CAD build for the part. Positions are in the model's coordinates, mm. A direction names the side the tool comes from. Coordinates: 2 decimals unless noted, no trailing zeros. Order: outer loops, then holes, each group sorted by start corner. A loop starts at its lowest first (then second) coordinate and runs counter-clockwise, first axis right, second up. Notation, with made-up numbers: (27.5, -30.5) - (83.5, -30.5) arc R19 ccw to (83.5, -5.5) - close; hole circle Ø3 at (-14, 84). An arc over 180 degrees is marked (long way). Return JSON: item names as keys, results as strings.
from build123d import *

# Parameters (mm, degrees)
F1_DEPTH = 88.9
F2_SIZE  = 5.08
F3_SIZE  = 5.08
F4_SIZE  = 5.08
F5_SIZE  = 5.08
F6_SIZE  = 5.08
F7_SIZE  = 5.08
F8_R     = 8.414365
F9_DEPTH = 101.6
F10_SIZE = 7.62


with BuildPart() as f1:
    # F0 (on Front) → F1 (new body)
    with BuildSketch(Plane.XZ):
        Polygon((-22.467206, -10.215149), (2.772436, -24.524237), (24.180665, -4.941663), (12.172037, 21.470121), (-16.657933, 18.210928), align=None)
    extrude(amount=F1_DEPTH)

    # F2
    f2_edges = [f1.edges().sort_by_distance(p)[0] for p in [
        (-9.847385, -88.9, -17.369693),
    ]]
    chamfer(f2_edges, length=F2_SIZE)

    # F3
    f3_edges = [f1.edges().sort_by_distance(p)[0] for p in [
        (-19.027823, -88.9, 6.614521),
    ]]
    chamfer(f3_edges, length=F3_SIZE)

    # F4
    f4_edges = [f1.edges().sort_by_distance(p)[0] for p in [
        (0.410862, -88.9, 20.140535),
    ]]
    chamfer(f4_edges, length=F4_SIZE)

    # F5
    f5_edges = [f1.edges().sort_by_distance(p)[0] for p in [
        (19.28175, -88.9, 5.833014),
    ]]
    chamfer(f5_edges, length=F5_SIZE)

    # F6
    f6_edges = [f1.edges().sort_by_distance(p)[0] for p in [
        (13.476551, -88.9, -14.73295),
    ]]
    chamfer(f6_edges, length=F6_SIZE)

    # F7
    f7_edges = [f1.edges().sort_by_distance(p)[0] for p in [
        (-19.562569, 0, 3.997889),
        (-2.242948, 0, 19.840525),
        (18.176351, 0, 8.264229),
        (13.476551, 0, -14.73295),
        (-9.847385, 0, -17.369693),
    ]]
    chamfer(f7_edges, length=F7_SIZE)

    # F8 (on face) → F9 (join)
    with BuildSketch(Plane.XZ.offset(88.9)):
        Circle(F8_R)
    extrude(amount=F9_DEPTH)

    # F10
    f10_edges = [f1.edges().sort_by_distance(p)[0] for p in [
        (-8.414365, -190.5, 0),
    ]]
    chamfer(f10_edges, length=F10_SIZE)


solid = f1.part
Item 1: Drop flat-ended pins along their axis: P1, Ø1, axis at x = -6.5, y = -32, coming from the -Z side; P2, Ø12, axis at x = -10, z = 6, coming from the -Y side; P3, Ø6, axis at x = 15.5, z = 2.5, coming from the -Y side. Give the stop position or say it passes through.
Findings below:
{"P1": "stops at z = -19.55", "P2": "stops at y = -185.63", "P3": "stops at y = -88.9"}
Item 2: Band-saw the part on A-A, the plane y = -127.5. List the corners of the cut face in (x, z), then the cut area to 3 significant figures.
Findings below:
{"outline": "circle Ø16.83 at (0, 0)", "area": "222 mm²"}
Item 3: Band-saw the part on B-B, the plane y = -28. List the corners of the cut face in (x, z), then the cut area to 3 significant figures.
Findings below:
{"outline": "(-22.47, -10.22) - (2.77, -24.52) - (24.18, -4.94) - (12.17, 21.47) - (-16.66, 18.21) - close", "area": "1,450 mm²"}
Item 4: Which spindle directions (+Z, -Z, +X, -X, +Y, -Y) get a long thin tool onto all of the face, cutting with end or side? Do faces 1 (the flat face through (-17.07, -2.58, 3.7)), 2 (the cylindrical face through (4.524, -135.232, 7.095)). Say none if no direction does.
Findings below:
{"face 1": "+Z, -X, +Y", "face 2": "-Y"}
Item 5: Wall check: L1, parallel to Y at x = -0.5, z = -14; L2, parallel to Y at x = -7, z = -2; L3, parallel to X at y = -92, z = 5. Give the ranges that are in metal, low to high. Write a range as [from, to].
Findings below:
{"L1": "y = [-88.9, 0]", "L2": "y = [-184.01, 0]", "L3": "x = [-6.77, 6.77]"}
